Answer from the drawing. Dimensions are ordinates in mm from the lowest x, y and z of the part. Round coordinates to 2 decimals unless told otherwise and drop trailing zeros. Loops run counter-clockwise (first coordinate to the right, second up) from the corner with the lowest first, then second, coordinate; pieces in that order, holes last. Notation, with made-up numbers: (66.25, -17.75) - (90.25, -17.75) arc R15 cw to (90.25, 2.25) - close; hole circle Ø10 at (57, -25.75). An arc over 180 degrees is marked (long way). Return JSON: item names as keys, results as strings.
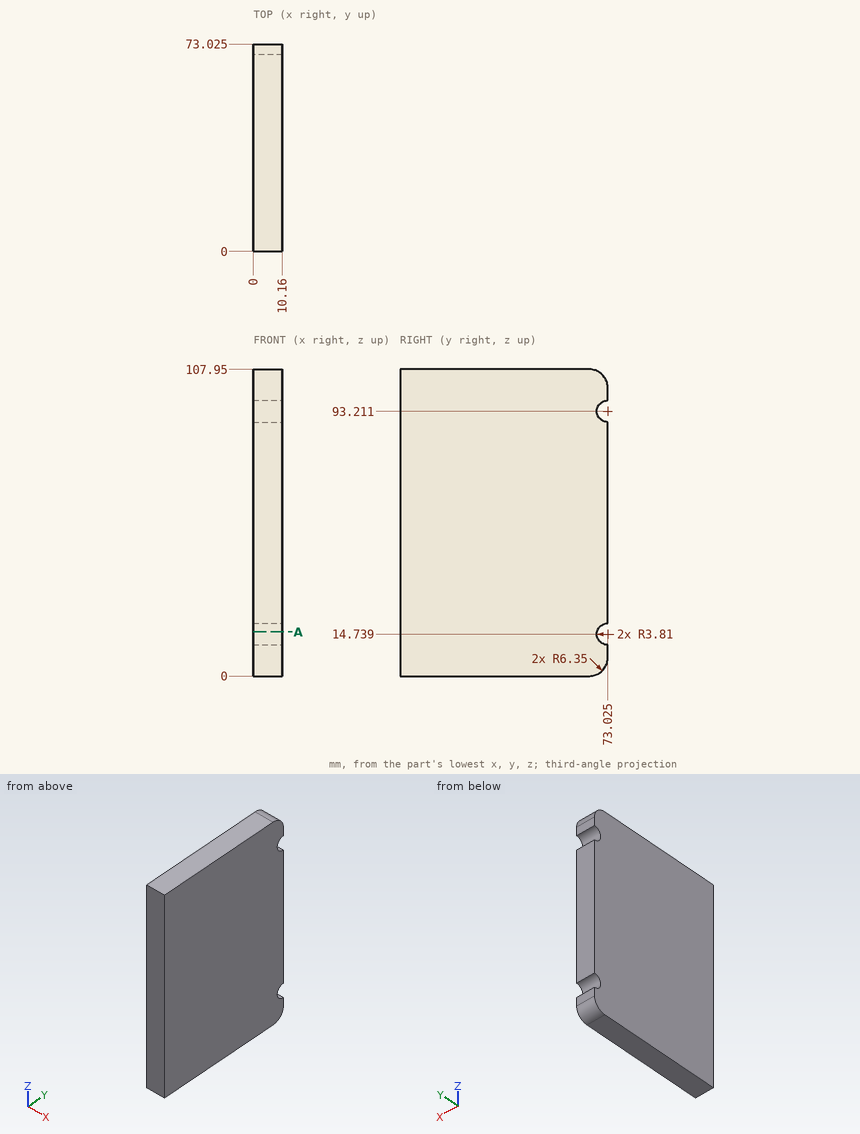
1) Find the intervals of material crossed by L1, parallel to Y at x = 7.5, z = 96; L2, parallel to Y at x = 9.25, z = 11.5, in increasing order.
Verdict:
{"L1": "y = 0 to 70.43", "L2": "y = 0 to 71.02"}
2) Section A-A (z = 15.5) is taken. Give the vertices of the cut face in (x, y), and give its area (3 significant figures).
Verdict:
{"outline": "(0, 0) - (10.16, 0) - (10.16, 69.29) - (0, 69.29) - close", "area": "704 mm2"}
3) A flat-ended cylindrical pin translates along its axis: pin 1 (2 mm diameter, centred on y = 27.5, z = 51.5, fed in from -X). Find the tip coordinate at first contact, or state that the pin passes through.
Verdict:
{"pin 1": "stops at x = 0"}
